from build123d import *

# Parameters (mm, degrees)
F0_W     = 78
F0_H     = 38
F0_R     = 2.25
F0_R_2   = 6.5
F1_DEPTH = 4
F2_R     = 5


# Not quite as in the source:
# - a feature names something its author has since deleted; it is built from what else it names


with BuildPart() as f1:
    # F0 (on Top) → F1 (new body)
    with BuildSketch(Plane.XY):
        Rectangle(F0_W, F0_H)
        with Locations((-29, -13)):
            Circle(F0_R, mode=Mode.SUBTRACT)
        with Locations((-13, -13)):
            Circle(F0_R, mode=Mode.SUBTRACT)
        with Locations((13, -13)):
            Circle(F0_R, mode=Mode.SUBTRACT)
        with Locations((29, -13)):
            Circle(F0_R, mode=Mode.SUBTRACT)
        with Locations((-29, 13)):
            Circle(F0_R, mode=Mode.SUBTRACT)
        with Locations((-13, 13)):
            Circle(F0_R, mode=Mode.SUBTRACT)
        Circle(F0_R_2, mode=Mode.SUBTRACT)
        with Locations((13, 13)):
            Circle(F0_R, mode=Mode.SUBTRACT)
        with Locations((29, 13)):
            Circle(F0_R, mode=Mode.SUBTRACT)
    extrude(amount=-F1_DEPTH)

    # F2
    f2_edges = [f1.edges().sort_by_distance(p)[0] for p in [
        (-39, -19, -2),
        (39, -19, -2),
        (39, 19, -2),
        (-39, 19, -2),
    ]]
    fillet(f2_edges, radius=F2_R)


solid = f1.part
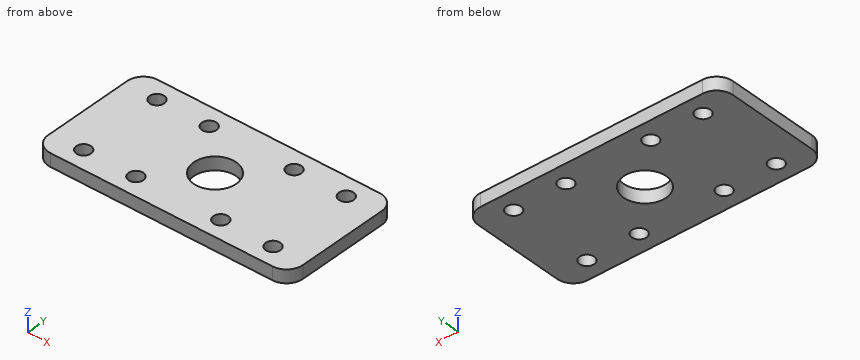
Source: CAD feature listing. Evaluate the final solid. Frame: model axes, mm. Round coordinates to 2 decimals unless told otherwise and drop trailing zeros. Loops run counter-clockwise (first coordinate to the right, second up) from the corner with the lowest first, then second, coordinate; pieces in that order, holes last. Notation, with made-up numbers: M -16.75,79 L 37.25,79 A24 cw 37.25,111 Z; hole C 81,-18 d9. An arc over 180 degrees is marked long. Return JSON: item names as keys, results as strings. Group by question number.
1. Section query B-B on x = 0. Output: boundary loops of the cut face in (y, z), and give its area (3 significant figures).
2. Section query A-A on x = -13. Output: boundary loops of the cut face in (y, z), and give its area (3 significant figures).
3. Material intervals for line 1 along Y through (x, z) = (29, -1.6); line 2 along X through (y, z) = (-14.5, -1.1); line 3 along X through (y, z) = (-12, -0.2), sorted ascending. Write a range as from..to.
4. Section query D-D on z = -1.5. State how many separate pieces and enclosed holes the cut face has, and give its area (3 significant figures).
5. Section query C-C on y = 13. Output: boundary loops of the cut face in (x, z).
Checks:
{
 "1": {"outline": "M -19,-4 L -6.5,-4 L -6.5,0 L -19,0 Z; M 6.5,-4 L 19,-4 L 19,0 L 6.5,0 Z", "area": "100 mm²"},
 "2": {"outline": "M -19,-4 L -15.25,-4 L -15.25,0 L -19,0 Z; M -10.75,-4 L 10.75,-4 L 10.75,0 L -10.75,0 Z; M 15.25,-4 L 19,-4 L 19,0 L 15.25,0 Z", "area": "116 mm²"},
 "3": {"line 1": "y = -19..-15.25, -10.75..10.75, 15.25..19", "line 2": "x = -38.97..-30.68, -27.32..-14.68, -11.32..11.32, 14.68..27.32, 30.68..38.97", "line 3": "x = -39..-31.02, -26.98..-15.02, -10.98..10.98, 15.02..26.98, 31.02..39"},
 "4": {"separate pieces": "1", "enclosed holes": "9", "area": "2,680 mm²"},
 "5": {"outline": "M -39,-4 L -31.25,-4 L -31.25,0 L -39,0 Z; M -26.75,-4 L -15.25,-4 L -15.25,0 L -26.75,0 Z; M -10.75,-4 L 10.75,-4 L 10.75,0 L -10.75,0 Z; M 15.25,-4 L 26.75,-4 L 26.75,0 L 15.25,0 Z; M 31.25,-4 L 39,-4 L 39,0 L 31.25,0 Z"}
}
